```python
from build123d import *

# Parameters (mm, degrees)
SKETCH1_R           = 4
BOSS_EXTRUDE1_DEPTH = 60


with BuildPart() as part:
    # Sketch1 → Boss-Extrude1 (new body)
    with BuildSketch(Plane.XY):
        Polygon((-78.477343622, -6.715827259), (-105.53442836, -6.715827259), (-105.53442836, -31.084686171), (-55.837306641, -31.084686171), (31.27656695, -31.084686171), (85.964626644, -31.084686171), (85.685037395, -6.772556192), (47.660564626, -6.772556192), (47.660564626, 67.701117608), (-78.477343622, 67.701117608), align=None)
        with Locations((-46.271365908, 61.586520729)):
            Circle(SKETCH1_R, mode=Mode.SUBTRACT)
        with Locations((21.710626217, 61.586520729)):
            Circle(SKETCH1_R, mode=Mode.SUBTRACT)
    extrude(amount=BOSS_EXTRUDE1_DEPTH)


solid = part.part
```
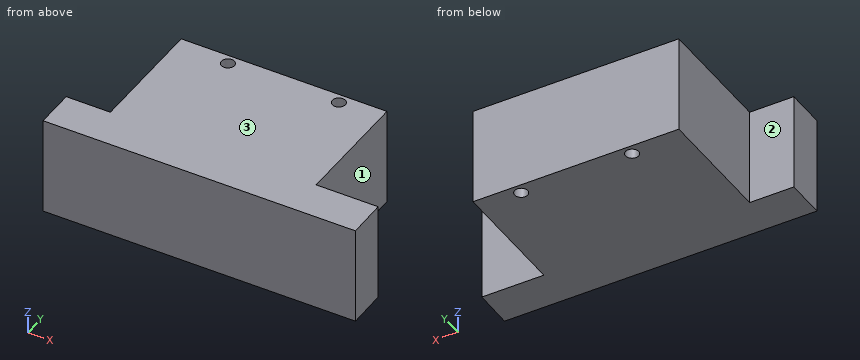
For this review, take the finished solid that the model builds, in its own axes (mm). Face numbers are marked on the shaded views. A direction names the side the tool comes from. Give positions to 0.01 mm unless a question says otherwise; leave off trailing zeros. Write each loop counter-clockwise with the first axis right and the second up, starting at its lowest first coordinate (ties: lowest second). Pieces come first, ordered by that corner, then holes. Notation, with made-up numbers: M 12.5,3 L 54.5,3 A29 ccw 54.5,26 Z; hole C -21.5,-38 d3. An arc over 180 degrees is marked long. One line per item, written item: value.
1) Take a section at C-C, the plane y = 24. Write out the cut boundary in (x, z), then the cut area to 3 significant figures.
Results are:
outline: M -78.48,0 L 47.66,0 L 47.66,60 L -78.48,60 Z
area: 7,570 mm²
2) For line 1 (X direction, y = 58.5, z = 38.5); line 2 (X direction, y = 21.5, z = 8); line 3 (X direction, y = -9, z = 15), list the stretches that pass through material, from the lowest coordinate up. Write a range as from..to.
Results are:
line 1: x = -78.48..-48.82, -43.73..19.17, 24.25..47.66
line 2: x = -78.48..47.66
line 3: x = -105.53..85.71
3) Take a section at B-B, the plane x = 60. Write out the cut boundary in (y, z).
Results are:
outline: M -31.08,0 L -6.77,0 L -6.77,60 L -31.08,60 Z
4) Take a section at A-A, the plane z = 50.5. Write out the cut boundary in (x, y).
Results are:
outline: M -105.53,-31.08 L 85.96,-31.08 L 85.69,-6.77 L 47.66,-6.77 L 47.66,67.7 L -78.48,67.7 L -78.48,-6.72 L -105.53,-6.72 Z; hole C -46.27,61.59 d8; hole C 21.71,61.59 d8
5) For P1, Ø6, axis at y = 40.5, z = 17, coming from the -X side; P2, Ø8, axis at x = -96, z = 19.5, coming from the +Y side, all flat-tipped, find the tip position at first contact; note any pin that passes through.
Results are:
P1: stops at x = -78.48
P2: stops at y = -6.72
6) For the marked faces 1, 2 and 3, list the 3-axis set-ups (+Z, -Z, +X, -X, +Y, -Y) from which the entire face can be reached by the end or side of a thin tool; tool diameter is ignored.
Results are:
face 1: +Z, -Z, +X, +Y
face 2: +Z, -Z, -X, +Y
face 3: +Z, +X, -X, +Y, -Y
